The model under review builds one solid part; all positions refer to its coordinate system, in mm. A direction names the side the tool comes from. Round coordinates to 2 decimals unless told otherwise and drop trailing zeros. Loops run counter-clockwise (first coordinate to the right, second up) from the corner with the lowest first, then second, coordinate; pieces in that order, holes last. Notation, with made-up numbers: M 47.5,14 L 87.5,14 A11 ccw 87.5,27 Z; hole C 30.25,29.25 d5. An arc over 180 degrees is marked long. Return JSON: item names as keys, results as strings. Group by question number.
Q1. For faces 4 (the face through (72.46, -61.77, 12.51)), 5 (the face through (0, -123, 50)), 6 (the face through (1, -120, 27)), 7 (the face through (10.459, -122.535, 32.932)), list the 3-axis set-ups (+Z, -Z, +X, -X, +Y, -Y) from which the entire face can be reached by the end or side of a thin tool; tool diameter is ignored.
Q2. To check wall thickness, follow line 1 along Y through (x, z) = (72.7, 37.5); line 2 along X through (y, z) = (47.5, 11); line 3 along Y through (x, z) = (69.5, 48). State the ranges of each line that lie inside material, in increasing order.
Q3. Consider section A-A (z = 25). Count the separate pieces of the cut face and the enclosed holes in it, and give its area (3 significant figures).
Q4. Clearance check with flat-ended pins moving along their axes: pin 1 Ø12.5 at (x, y) = (-37, 103.5) entering from +Z; pin 2 Ø1.5 at (x, y) = (72.5, 12.5) entering from +Z. State where each tip first meets the part, or that it passes through.
Q5. Consider section D-D (z = 44.5). State the section outline as (x, y) points.
Q6. Draft analysis for pull direction X (two halves, no side actions). For faces 1 (the face through (-1, 120, 27)), 2 (the face through (75, 2, 19)), 3 (the face through (0, 121, 50)), state which applies: pulls with the +X half, pulls with the -X half, needs draft (parallel to the pull), parting line crosses it, or undercut.
Q7. Consider section B-B (x = -8.5). State the section outline as (y, z) points, and give its area (3 significant figures).
Q8. Consider section C-C (y = 96). State the section outline as (x, z) points.
Autodesk Inventor part; units mm, degrees
ref_plane "YZ Plane" through (0, 0, 0) normal (1, 0, 0) x (0, 1, 0)
ref_plane "XZ Plane" through (0, 0, 0) normal (0, 1, 0) x (-1, 0, 0)
ref_plane "XY Plane" through (0, 0, 0) normal (0, 0, 1) x (1, 0, 0)
sketch "Sketch1" plane through (0, 0, 0) normal (0, 0, 1) x (1, 0, 0)
  line L0 (-75, 125) -> (75, 125)
  line L1 (75, 125) -> (75, -125)
  line L2 (75, -125) -> (-75, -125)
  line L3 (-75, -125) -> (-75, 125)
  line L4 (-75, 125) -> (75, -125) construction
  line L5 (75, 125) -> (-75, -125) construction
  point P0 (0, 0)
  dimension "d0" = 150
  dimension "d1" = 250
extrude "Extrusion1" add sketch "Sketch1" along normal blind 50
shell "Shell1" thickness 5 removed faces 1 at (-25, -41.6667, 50)
sketch "Sketch2" plane through (-75, -125, 0) normal (0, -1, 0) x (1, 0, 0)
  line L0 (75, 0) -> (75, 50)
  line L1 (150, 50) -> (0, 50)
  line L2 (52.5, 35) -> (97.5, 35)
  line L3 (97.5, 35) -> (97.5, 15)
  line L4 (97.5, 15) -> (52.5, 15)
  line L5 (52.5, 15) -> (52.5, 35)
  line L6 (52.5, 35) -> (97.5, 15) construction
  line L7 (97.5, 35) -> (52.5, 15) construction
  line L8 (97.5, 25) -> (94.5, 25)
  line L9 (94.5, 25) -> (78.5, 25)
  line L10 (52.5, 25) -> (55.5, 25)
  line L11 (55.5, 25) -> (71.5, 25)
  circle A0 centre (86.5, 25) radius 8
  circle A1 centre (63.5, 25) radius 8
  point P0 (75, 25)
  dimension "d5" = 45
  dimension "d6" = 20
  dimension "d7" = 3
  dimension "d8" = 16
  dimension "d9" = 3
  dimension "d10" = 16
  dimension "d11" = 16
  dimension "d12" = 16
extrude "Extrusion2" cut sketch "Sketch2" against normal blind 86 contours A1 L11 | L11 A1 | A0 L9 | L9 A0
sketch "Sketch3" plane through (-75, -125, 0) normal (-1, 0, 0) x (0, 0, 1)
  line L0 (0, 125) -> (50, 125)
  line L1 (50, 5) -> (50, 245)
  line L2 (25, 125) -> (25, 0)
  line L3 (0, 0) -> (50, 0)
  line L4 (25, 62.5) -> (50, 62.5)
  circle A0 centre (37.5, 62.5) radius 25
  dimension "d15" = 50
extrude "Extrusion3" cut sketch "Sketch3" against normal blind 192.25 contours A0 L1 L4 L2 | L2 A0 | A0 L1 | L4 L1 A0 L2
sketch "Sketch4" plane through (-75, -125, 0) normal (-1, 0, 0) x (0, 0, 1)
  line L0 (0, 125) -> (50, 125)
  line L1 (50, 245) -> (50, 84.1506)
  line L2 (25, 125) -> (25, 250)
  line L3 (0, 250) -> (50, 250)
  line L4 (25, 187.5) -> (50, 187.5)
  circle A0 centre (37.5, 187.5) radius 25
  dimension "d18" = 50
extrude "Extrusion4" cut sketch "Sketch4" against normal blind 216.5 contours A0 L2 | L2 L4 L1 A0 | L1 A0 | L2 A0 L1 L4
sketch "Sketch5" plane through (0, 0, 50) normal (0, 0, 1) x (1, 0, 0)
  line L0 (-75, 40.8494) -> (-75, -40.8494)
  line L1 (-75, 0) -> (-70, 0)
  line L2 (-70, -40.8494) -> (-70, 40.8494)
  circle A0 centre (-72.5, 0) radius 1.25
  point P0 (0, 0)
  dimension "d21" = 2.5
extrude "Extrusion5" add sketch "Sketch5" along normal blind 2.75
sketch "Sketch6" plane through (0, 0, 50) normal (0, 0, 1) x (1, 0, 0)
  line L0 (70, 40.8494) -> (70, -40.8494)
  line L1 (70, 0) -> (75, 0)
  line L2 (75, -125) -> (75, 125)
  circle A0 centre (72.5, 0) radius 1.25
  point P0 (0, 0)
  dimension "d24" = 2.5
extrude "Extrusion6" add sketch "Sketch6" along normal blind 2.75
sketch "Sketch7" plane through (75, -125, 0) normal (1, 0, 0) x (0, 0, -1)
  point P0 (0, 125)
properties part number "broomba top"
Values:
{
 "1": {"face 4": "+X, -X", "face 5": "+Z, +X, -X, -Y", "face 6": "+Z", "face 7": "-Y"},
 "2": {"line 1": "y = -125 to -87.5, -37.5 to 37.5, 87.5 to 125", "line 2": "x = -75 to -70, 70 to 75", "line 3": "y = -125 to -120, 120 to 125"},
 "3": {"separate pieces": "6", "enclosed holes": "0", "area": "2,870 mm2"},
 "4": {"pin 1": "stops at z = 5", "pin 2": "stops at z = 50"},
 "5": {"outline": "M -75,-125 L 75,-125 L 75,-86.5 L 70,-86.5 L 70,-120 L -70,-120 L -70,-86.5 L -75,-86.5 Z; M -75,-38.5 L -70,-38.5 L -70,38.5 L -75,38.5 Z; M -75,86.5 L -70,86.5 L -70,120 L 70,120 L 70,86.5 L 75,86.5 L 75,125 L -75,125 Z; M 70,-38.5 L 75,-38.5 L 75,38.5 L 70,38.5 Z"},
 "6": {"face 1": "undercut", "face 2": "pulls with the +X half", "face 3": "needs draft"},
 "7": {"outline": "M -125,0 L 125,0 L 125,50 L 120,50 L 120,5 L -120,5 L -120,17.58 L -125,17.58 Z; M -125,32.42 L -120,32.42 L -120,50 L -125,50 Z", "area": "1,630 mm2"},
 "8": {"outline": "M -75,0 L 75,0 L 75,50 L 70,50 L 70,5 L -70,5 L -70,50 L -75,50 Z"}
}
